```python
from build123d import *

# Parameters (mm, degrees)
F_01_START                  = -1.8
S01_LOW_PROFILE_HEAD_R      = 2.55
F_01_LOW_PROFILE_HEAD_DEPTH = 1.8
S02_SMOOTH_JOURNAL_R        = 1.5
F_02_SMOOTH_JOURNAL_DEPTH   = 13.1
F_03_START                  = 13.1
S03_M3_THREADED_TIP_R       = 1.48
F_03_M3_THREADED_TIP_DEPTH  = 4.18
F_04_START                  = -1.9
F_04_HEX_SOCKET_DEPTH       = 1.05


with BuildPart() as part:
    # S01 - Low profile head → 01 - Low profile head (new body)
    with BuildSketch(Plane.XY.offset(F_01_START)):
        Circle(S01_LOW_PROFILE_HEAD_R)
    extrude(amount=F_01_LOW_PROFILE_HEAD_DEPTH)

    # S02 - Smooth journal → 02 - Smooth journal (add)
    with BuildSketch(Plane.XY):
        with Locations(Location((0, 0, 0), (0, 0, 180))):
            Circle(S02_SMOOTH_JOURNAL_R)
    extrude(amount=F_02_SMOOTH_JOURNAL_DEPTH)

    # S03 - M3 threaded tip → 03 - M3 threaded tip (add)
    with BuildSketch(Plane.XY.offset(F_03_START)):
        Circle(S03_M3_THREADED_TIP_R)
    extrude(amount=F_03_M3_THREADED_TIP_DEPTH)

    # S04 - Hex socket → 04 - Hex socket (cut)
    with BuildSketch(Plane.XY.offset(F_04_START)):
        Polygon((0.995929214, 0.575), (0, 1.15), (-0.995929214, 0.575), (-0.995929214, -0.575), (0, -1.15), (0.995929214, -0.575), align=None)
    extrude(amount=F_04_HEX_SOCKET_DEPTH, mode=Mode.SUBTRACT)


solid = part.part
```
The listing builds one solid part. Answer for the finished solid, in the listing's coordinates (mm). A direction names the side the tool comes from. Round coordinates to 2 decimals unless told otherwise and drop trailing zeros. Write each loop counter-clockwise with the first axis right and the second up, starting at its lowest first coordinate (ties: lowest second). Pieces come first, ordered by that corner, then holes. Notation, with made-up numbers: (18.25, 14) -> (32.25, 14) arc R19 cw to (32.25, 20) -> close; hole circle Ø10 at (58, -10.5). An arc over 180 degrees is marked (long way). Use CSV: the item, a comma, the result in double quotes. Start each with the question number.
(1) Consider L1, parallel to Z at x = -0.95, y = 1.5; L2, parallel to Z at x = 0.8, y = 0.05; L3, parallel to X at y = 0.05, z = 2. Determine where each line is inside the solid, lowest interval first. Write a range as from..to.
(2) Which of the six approach directions +Z, -Z, +X, -X, +Y, -Y give full straight-line access (tool end or side, diameter ignored) to faces 1 (the face through (-0.491, 0.867, -1.332)), 2 (the face through (-1.174, -0.901, 15.161)), 3 (the face through (0, 0, 17.28))?
(3) Each of these flat-tipped pins is pushed along its axis until it touches: pin 1 (3 mm diameter, centred on x = 1.5, z = 7, fed in from +Y); pin 2 (3 mm diameter, centred on x = -0.5, z = 13, fed in from -Y); pin 3 (1 mm diameter, centred on x = -1.5, z = 3.5, fed in from +Y). Where does it stop, or does it pass through?
(4) The mould has two halves that part along Y. Classify faces 4 (the face through (1, -1, -1.8)), 5 (the face through (-0.996, 0, -1)), 6 (the face through (1.18, -2.26, -0.91)): released by +Y, released by -Y, zero draft, split by the parting line, or undercut.
(5) Section B-B on z = 8.5 is taken. Give the vertices of the cut face in (x, y), then the cut area to 3 significant figures.
(6) Section D-D on z = 14.5 is taken. Give the vertices of the cut face in (x, y), then the cut area to 3 significant figures.
A:
1,L1,"z = -1.8..0"
1,L2,"z = -0.85..17.28"
1,L3,"x = -1.5..1.5"
2,face 1,"-Z"
2,face 2,"+Z"
2,face 3,"+Z, +X, -X, +Y, -Y"
3,pin 1,"stops at y = 1.5"
3,pin 2,"stops at y = -1.5"
3,pin 3,"stops at y = 1.12"
4,face 4,"zero draft"
4,face 5,"undercut"
4,face 6,"split by the parting line"
5,outline,"circle Ø3 at (0, 0)"
5,area,"7.07 mm²"
6,outline,"circle Ø2.96 at (0, 0)"
6,area,"6.88 mm²"
